Autodesk Inventor part; units mm, degrees
ref_plane "YZ Plane" through (0, 0, 0) normal (1, 0, 0) x (0, 1, 0)
ref_plane "XZ Plane" through (0, 0, 0) normal (0, 1, 0) x (-1, 0, 0)
ref_plane "XY Plane" through (0, 0, 0) normal (0, 0, 1) x (1, 0, 0)
sketch "Boceto1" plane through (0, 0, 0) normal (0, 1, 0) x (-1, 0, 0)
  circle A0 centre (0, 0) radius 4.5
  dimension "d0" = 9
extrude "Extrusión1" add sketch "Boceto1" along normal blind 87
fillet "Empalme1" radius 4.5 1 edges at (4.5, 87, 0)
sketch "Boceto2" plane through (0, 0, 0) normal (0, -1, 0) x (1, 0, 0)
  circle A0 centre (0, 0) radius 4.5
  circle A1 centre (0, 0) radius 4.5
  line L0 (3.8723, -2.2357) -> (3.8971, -2.25)
  line L1 (0, 0) -> (5.1962, 0) construction
  line L2 (4.5, -2.5981) -> (4.5, 2.5981)
  line L3 (0, 0) -> (5.1962, 0) construction
  line L4 (4.5, 2.5981) -> (0, 5.1958)
  line L5 (0, 5.1958) -> (-4.5, 2.5981)
  line L6 (-4.5, 2.5981) -> (-4.5409, -2.5978)
  line L7 (-4.5409, -2.5978) -> (-0.0409, -5.1955)
  line L8 (-0.0409, -5.1955) -> (4.5, -2.5981)
  dimension "d9" = 30
  dimension "d11" = 5.196
  dimension "d12" = 5.196
  dimension "d13" = 5.196
  dimension "d14" = 5.196
extrude "Extrusión2" [suppressed]
ref_plane "Plano de trabajo1" through (-2.2861, 0, 1.3081) normal (-0.5, 0, -0.8661) x (-0.8661, 0, 0.5)
ref_plane "Plano de trabajo2" through (4.5, 0, -2.5981) normal (0.5, 0, 0.866) x (0, 1, 0)
sketch "Boceto4" plane through (0, 0, 0) normal (1, 0, 0) x (0, 1, 0)
  circle A0 centre (4.5, 0) radius 4.5
  line L0 (0, -4.5) -> (0, 4.5)
  line L1 (0, 4.5) -> (82.5, 4.5)
  point P0 (0, 0)
  dimension "d18" = 9
  dimension "d19" = 4.5
  dimension "d20" = 4.5
extrude "Extrusión3" add sketch "Boceto4" along normal blind 24.5 contours A0
sketch "Boceto5" plane through (24.5, 4.5, 0) normal (1, 0, 0) x (0, 0, -1)
  circle A0 centre (0, 0) radius 4.5
  circle A1 centre (0, 0) radius 4.5
  line L0 (0, 4.5) -> (-2.5981, 4.5)
  line L1 (-2.5981, 4.5) -> (2.5981, 4.5)
  line L2 (0, 4.5) -> (2.5981, 4.5) construction
  line L3 (0, 0) -> (5.9241, 0) construction
  line L4 (0, 0) -> (-9, 0)
  line L5 (0, 0) -> (6.2143, 0) construction
  line L6 (-3.8971, 2.25) -> (-5.1962, 0)
  line L7 (-5.1962, 0) -> (-2.5981, 4.5)
  line L8 (-5.1962, 0) -> (-2.5981, -4.5)
  line L9 (-5.1962, 0) -> (2.2031, 0) construction
  line L10 (4.5, -4.5) -> (-4.5, -4.5)
  line L11 (0, -4.5) -> (-2.5981, -4.5)
  line L12 (-4.5, -4.5) -> (2.5981, -4.5)
  line L13 (0, -4.5) -> (2.5981, -4.5)
  line L14 (2.5981, -4.5) -> (5.1096, -0.1499)
  line L15 (5.1096, -0.1499) -> (5.1962, 0)
  line L16 (5.1962, 0) -> (2.5981, 4.5)
  line L17 (5.1962, 0) -> (10.3923, 0) construction
  line L18 (-2.5981, -4.5) -> (-5.1962, 0)
  line L19 (-2.5981, 4.5) -> (2.5981, 4.5)
  dimension "d26" = 60
  dimension "Q" = 2.5981
  dimension "d28" = 2.5981
  dimension "d29" = 120
extrude "Extrusión4" add sketch "Boceto5" along normal blind 12
equation "\"d28\" = Q"
properties part number "antena"
Source: CAD feature listing. Evaluate the final solid. Frame: model axes, mm. A direction names the side the tool comes from. Give positions to 0.01 mm unless a question says otherwise; leave off trailing zeros. Write each loop counter-clockwise with the first axis right and the second up, starting at its lowest first coordinate (ties: lowest second). Pieces come first, ordered by that corner, then holes. Notation, with made-up numbers: M 7.25,82 L 49.25,82 A13 ccw 49.25,102 Z; hole C -19.75,3.25 d9. An arc over 180 degrees is marked long. Return JSON: item names as keys, results as strings. Group by question number.
1) Cut plane C-C, the plane y = 28. Output: boundary loops of the cut face in (x, z), then the cut area to 3 significant figures.
2) First-contact query: pin 1 Ø8 at (x, y) = (2, 23) entering from -Z; pin 2 Ø1.5 at (y, z) = (22.5, 3.5) entering from -X; pin 3 Ø2.5 at (y, z) = (5, -3) entering from -X. Flat tips, straight axial feed; report the tip coordinate or a pass-through.
3) Cut plane D-D, the plane x = 10.5. Output: boundary loops of the cut face in (y, z), then the cut area to 3 significant figures.
4) Cut plane B-B, the plane z = -1. Output: boundary loops of the cut face in (x, y).
5) Set-up query: faces 4 (the face through (30.416, 6.718, -3.915)), 5 (the face through (30, 9, 0)), 6 (the face through (24.5, 0.5, -2.4)). Return all of +Z, -Z, +X, -X, +Y, -Y with unobstructed straight access to the full face (end or side cutting, diameter ignored); none if empty.
6) Draft query along X for faces 1 (the face through (24.5, 8.5, 2.4)), 2 (the face through (36.5, 5, 0)), 3 (the face through (30, 0, 0)). Return one class per face: released by +X, released by -X, zero draft, split by the parting line, or undercut.
7) Ray query, L1, parallel to X at y = 32, z = -2.25; L2, parallel to X at y = 76, z = 0; L3, parallel to Y at x = 31.5, z = -1.5. Return the intervals inside material, ascending.
8) Cut plane A-A, the plane x = 27. Output: boundary loops of the cut face in (y, z), then the cut area to 3 significant figures.
Data:
{
 "1": {"outline": "C 0,0 d9", "area": "63.6 mm²"},
 "2": {"pin 1": "stops at z = -4.5", "pin 2": "stops at x = -3.56", "pin 3": "stops at x = -4.15"},
 "3": {"outline": "C 4.5,0 d9", "area": "63.6 mm²"},
 "4": {"outline": "M -4.39,0 L 4.39,0 L 4.39,0.11 L 24.5,0.11 L 24.5,0 L 36.5,0 L 36.5,9 L 24.5,9 L 24.5,8.89 L 4.39,8.89 L 4.39,82.5 A4.39 ccw -4.39,82.5 Z"},
 "5": {"face 4": "-Z, +X, +Y", "face 5": "+Z, -Z, +X, +Y", "face 6": "-Z, -Y"},
 "6": {"face 1": "undercut", "face 2": "released by +X", "face 3": "zero draft"},
 "7": {"L1": "x = -3.9 to 3.9", "L2": "x = -4.5 to 4.5", "L3": "y = 0 to 9"},
 "8": {"outline": "M 0,-2.6 L 4.35,-5.11 L 4.5,-5.2 L 9,-2.6 L 9,2.6 L 6.75,3.9 L 4.5,5.2 L 0,2.6 Z", "area": "70.1 mm²"}
}
